```python
from build123d import *

# Parameters (mm, degrees)
F1_DEPTH = 12.7


with BuildPart() as f1:
    # F0 (on Top) → F1 (new body)
    with BuildSketch(Plane.XY):
        Polygon((6.17555, -62.701412), (18.289327, -60.291831), (16.85737, -55.571301), (5.692037, -57.792224), align=None)
        Polygon((-44.890152, -36.840395), (-48.703367, -39.96982), (-39.96982, -48.703367), (-36.840395, -44.890152), align=None)
        Polygon((-55.571301, -16.85737), (-60.291831, -18.289327), (-55.56527, -29.700256), (-51.214805, -27.374883), align=None)
        Polygon((5.692037, 57.792224), (-5.692037, 57.792224), (-16.85737, 55.571301), (-27.374883, 51.214805), (-36.840395, 44.890152), (-44.890152, 36.840395), (-51.214805, 27.374883), (-55.571301, 16.85737), (-57.792224, 5.692037), (-57.792224, -5.692037), (-55.571301, -16.85737), (-51.214805, -27.374883), (-44.890152, -36.840395), (-36.840395, -44.890152), (-27.374883, -51.214805), (-16.85737, -55.571301), (-5.692037, -57.792224), (5.692037, -57.792224), (16.85737, -55.571301), (27.374883, -51.214805), (36.840395, -44.890152), (44.890152, -36.840395), (51.214805, -27.374883), (55.571301, -16.85737), (57.792224, -5.692037), (57.792224, 5.692037), (55.571301, 16.85737), (51.214805, 27.374883), (44.890152, 36.840395), (36.840395, 44.890152), (27.374883, 51.214805), (16.85737, 55.571301), align=None)
        Polygon((62.701412, -6.17555), (62.701412, 6.17555), (57.792224, 5.692037), (57.792224, -5.692037), align=None)
        Polygon((60.291831, -18.289327), (62.701412, -6.17555), (57.792224, -5.692037), (55.571301, -16.85737), align=None)
        Polygon((-27.374883, -51.214805), (-29.700256, -55.56527), (-18.289327, -60.291831), (-16.85737, -55.571301), align=None)
        Polygon((55.56527, -29.700256), (60.291831, -18.289327), (55.571301, -16.85737), (51.214805, -27.374883), align=None)
        Polygon((18.289327, 60.291831), (6.17555, 62.701412), (5.692037, 57.792224), (16.85737, 55.571301), align=None)
        Polygon((29.700256, 55.56527), (18.289327, 60.291831), (16.85737, 55.571301), (27.374883, 51.214805), align=None)
        Polygon((-57.792224, 5.692037), (-62.701412, 6.17555), (-62.701412, -6.17555), (-57.792224, -5.692037), align=None)
        Polygon((-57.792224, -5.692037), (-62.701412, -6.17555), (-60.291831, -18.289327), (-55.571301, -16.85737), align=None)
        Polygon((-36.840395, 44.890152), (-39.96982, 48.703367), (-48.703367, 39.96982), (-44.890152, 36.840395), align=None)
        Polygon((-27.374883, 51.214805), (-29.700256, 55.56527), (-39.96982, 48.703367), (-36.840395, 44.890152), align=None)
        Polygon((48.703367, 39.96982), (39.96982, 48.703367), (36.840395, 44.890152), (44.890152, 36.840395), align=None)
        Polygon((-16.85737, 55.571301), (-18.289327, 60.291831), (-29.700256, 55.56527), (-27.374883, 51.214805), align=None)
        Polygon((-36.840395, -44.890152), (-39.96982, -48.703367), (-29.700256, -55.56527), (-27.374883, -51.214805), align=None)
        Polygon((39.96982, 48.703367), (29.700256, 55.56527), (27.374883, 51.214805), (36.840395, 44.890152), align=None)
        Polygon((29.700256, -55.56527), (39.96982, -48.703367), (36.840395, -44.890152), (27.374883, -51.214805), align=None)
        Polygon((-51.214805, -27.374883), (-55.56527, -29.700256), (-48.703367, -39.96982), (-44.890152, -36.840395), align=None)
        Polygon((-5.692037, -57.792224), (-6.17555, -62.701412), (6.17555, -62.701412), (5.692037, -57.792224), align=None)
        Polygon((48.703367, -39.96982), (55.56527, -29.700256), (51.214805, -27.374883), (44.890152, -36.840395), align=None)
        Polygon((18.289327, -60.291831), (29.700256, -55.56527), (27.374883, -51.214805), (16.85737, -55.571301), align=None)
        Polygon((39.96982, -48.703367), (48.703367, -39.96982), (44.890152, -36.840395), (36.840395, -44.890152), align=None)
        Polygon((6.17555, 62.701412), (-6.17555, 62.701412), (-5.692037, 57.792224), (5.692037, 57.792224), align=None)
        Polygon((-51.214805, 27.374883), (-55.56527, 29.700256), (-60.291831, 18.289327), (-55.571301, 16.85737), align=None)
        Polygon((55.56527, 29.700256), (48.703367, 39.96982), (44.890152, 36.840395), (51.214805, 27.374883), align=None)
        Polygon((-5.692037, 57.792224), (-6.17555, 62.701412), (-18.289327, 60.291831), (-16.85737, 55.571301), align=None)
        Polygon((-55.571301, 16.85737), (-60.291831, 18.289327), (-62.701412, 6.17555), (-57.792224, 5.692037), align=None)
        Polygon((60.291831, 18.289327), (55.56527, 29.700256), (51.214805, 27.374883), (55.571301, 16.85737), align=None)
        Polygon((62.701412, 6.17555), (60.291831, 18.289327), (55.571301, 16.85737), (57.792224, 5.692037), align=None)
        Polygon((-44.890152, 36.840395), (-48.703367, 39.96982), (-55.56527, 29.700256), (-51.214805, 27.374883), align=None)
        Polygon((-16.85737, -55.571301), (-18.289327, -60.291831), (-6.17555, -62.701412), (-5.692037, -57.792224), align=None)
    extrude(amount=F1_DEPTH)


solid = f1.part
```
Input: part model. Units: mm. Frame: model coordinates. Give positions to 0.01 mm unless a question says otherwise; leave off trailing zeros. Loops run counter-clockwise (first coordinate to the right, second up) from the corner with the lowest first, then second, coordinate; pieces in that order, holes last.
1) Line query: L1, parallel to X at y = -40, z = 3; L2, parallel to X at y = -26.5, z = 2; L3, parallel to Y at x = -44, z = 7.25. Output: solid intervals per line, ascending.
A:
L1: x = -48.67 to 48.67
L2: x = -56.89 to 56.89
L3: y = -44.67 to 44.67
2) Section query C-C on y = 46. Return the cut outline in (x, z), and give its area (3 significant figures).
A:
outline: (-42.67, 0) - (42.67, 0) - (42.67, 12.7) - (-42.67, 12.7) - close
area: 1,080 mm2
3) Contact query for flat-ended pins moving along their axis: pin 1 (3 mm diameter, centred on x = -9, z = 3.5, fed in from +Y); pin 2 (6 mm diameter, centred on x = -18.5, z = 8, fed in from +Y); pin 3 (2 mm diameter, centred on y = 28.5, z = 7.5, fed in from +X). Output: stop coordinate, or through.
A:
pin 1: stops at y = 62.44
pin 2: stops at y = 60.85
pin 3: stops at x = 56.48
4) Section query B-B on x = -47. Return the cut outline in (y, z), and give its area (3 significant figures).
A:
outline: (-41.67, 0) - (41.67, 0) - (41.67, 12.7) - (-41.67, 12.7) - close
area: 1,060 mm2
